from build123d import *

# Parameters (mm, degrees)
SKETCH1_W                        = 125
SKETCH1_H                        = 120
TEST_BASE_POSTION_DEPTH          = 11.215
SKETCH8_R                        = 20.5
FINGER_GEARS_DEPTH               = 7
SKETCH9_R                        = 10.5
INTERMEDIATE_GEAR_DEPTH          = 7
SKETCH11_R                       = 18.5
XL320_FINGER_KNUCKLE_MOUNT_DEPTH = 7
SKETCH10_R                       = 15.5
CONNECT_FINGER_HOLES_DEPTH       = 88.361468766
THUMB_MOUNT_HOLES_R              = 2.25
THUMB_MOUNT_HOLES_M4_DEPTH       = 88.361468766
SKETCH16_R                       = 2.25
FINGERS_MOUNT_HOLES_M4_DEPTH     = 88.361468766
SKETCH17_R                       = 3.25
CONNECT_HOLES_M6_DEPTH           = 88.361468766
NUTS_M4_DEPTH                    = 4
NUTS_M6_DEPTH                    = 6
SKETCH21_R                       = 1.5
FIX_GEAR_ROD_HOLE_DEPTH          = 2.5


with BuildPart() as part:
    # Sketch1 → Test_Base_Postion (new body)
    with BuildSketch(Plane(origin=(0, 0, 0), x_dir=(1, 0, 0), z_dir=(0, 1, 0))):
        Rectangle(SKETCH1_W, SKETCH1_H)
    extrude(amount=TEST_BASE_POSTION_DEPTH)

    # Sketch8 → Finger_Gears (cut)
    with BuildSketch(Plane(origin=(0, 11.215, 0), x_dir=(1, 0, 0), z_dir=(0, 1, 0))):
        with Locations((-25.25, -19)):
            Circle(SKETCH8_R)
        with Locations((-25.25, 19)):
            Circle(SKETCH8_R)
    extrude(amount=-FINGER_GEARS_DEPTH, mode=Mode.SUBTRACT)

    # Sketch9 → Intermediate_Gear (cut)
    with BuildSketch(Plane(origin=(0, 11.215, 0), x_dir=(1, 0, 0), z_dir=(0, 1, 0))):
        with Locations((0.646123438, -8.351488795)):
            Circle(SKETCH9_R)
    extrude(amount=-INTERMEDIATE_GEAR_DEPTH, mode=Mode.SUBTRACT)

    # Sketch11 → XL320_Finger_Knuckle_Mount (cut)
    with BuildSketch(Plane(origin=(0, 11.215, 0), x_dir=(1, 0, 0), z_dir=(0, 1, 0))):
        with Locations(Location((42, 0, 0), (0, 0, 270))):
            Circle(SKETCH11_R)
    extrude(amount=-XL320_FINGER_KNUCKLE_MOUNT_DEPTH, mode=Mode.SUBTRACT)

    # Sketch10 → Connect_Finger_Holes (cut, through all)
    with BuildSketch(Plane(origin=(0, 11.215, 0), x_dir=(1, 0, 0), z_dir=(0, 1, 0))):
        with Locations(Location((-25.25, 19, 0), (0, 0, 270))):
            Circle(SKETCH10_R)
        with Locations(Location((-25.25, -19, 0), (0, 0, 270))):
            Circle(SKETCH10_R)
        with Locations(Location((42, 0, 0), (0, 0, 270))):
            Circle(SKETCH10_R)
    extrude(amount=-CONNECT_FINGER_HOLES_DEPTH, mode=Mode.SUBTRACT)

    # Thumb_Mount_Holes → Thumb_Mount_Holes_(M4) (cut, through all)
    with BuildSketch(Plane(origin=(0, 11.215, 0), x_dir=(1, 0, 0), z_dir=(0, 1, 0))):
        with Locations(Location((21.5, 44.5, 0), (0, 0, 270))):
            Circle(THUMB_MOUNT_HOLES_R)
        with Locations(Location((42, 53.5, 0), (0, 0, 270))):
            Circle(THUMB_MOUNT_HOLES_R)
        with Locations(Location((48, -24, 0), (0, 0, 270))):
            Circle(THUMB_MOUNT_HOLES_R)
        with Locations(Location((36, -24, 0), (0, 0, 270))):
            Circle(THUMB_MOUNT_HOLES_R)
    extrude(amount=-THUMB_MOUNT_HOLES_M4_DEPTH, mode=Mode.SUBTRACT)

    # Sketch16 → Fingers_Mount_Holes_(M4) (cut, through all)
    with BuildSketch(Plane(origin=(0, 11.215, 0), x_dir=(1, 0, 0), z_dir=(0, 1, 0))):
        with Locations(Location((11.5, 41, 0), (0, 0, 270))):
            Circle(SKETCH16_R)
        with Locations(Location((11.5, -41, 0), (0, 0, 270))):
            Circle(SKETCH16_R)
        with Locations(Location((-53, 6, 0), (0, 0, 270))):
            Circle(SKETCH16_R)
        with Locations(Location((-53, -6, 0), (0, 0, 270))):
            Circle(SKETCH16_R)
    extrude(amount=-FINGERS_MOUNT_HOLES_M4_DEPTH, mode=Mode.SUBTRACT)

    # Sketch17 → Connect_Holes_(M6) (cut, through all)
    with BuildSketch(Plane(origin=(0, 11.215, 0), x_dir=(1, 0, 0), z_dir=(0, 1, 0))):
        with Locations(Location((-52.5, 50, 0), (0, 0, 270))):
            Circle(SKETCH17_R)
        with Locations(Location((-52.5, -50, 0), (0, 0, 270))):
            Circle(SKETCH17_R)
        with Locations(Location((52.5, -50, 0), (0, 0, 270))):
            Circle(SKETCH17_R)
    extrude(amount=-CONNECT_HOLES_M6_DEPTH, mode=Mode.SUBTRACT)

    # Sketch18 → Nuts_(M4) (cut)
    with BuildSketch(Plane.XZ):
        Polygon((11.5, 47.639528096), (5.75, 44.319764048), (5.75, 37.680235952), (11.5, 34.360471904), (17.25, 37.680235952), (17.25, 44.319764048), align=None)
        Polygon((11.5, -34.360471904), (5.75, -37.680235952), (5.75, -44.319764048), (11.5, -47.639528096), (17.25, -44.319764048), (17.25, -37.680235952), align=None)
        Polygon((15.75, -41.180235952), (15.75, -47.819764048), (21.5, -51.139528096), (27.25, -47.819764048), (27.25, -41.180235952), (21.5, -37.860471904), align=None)
        Polygon((42, -60.139528096), (47.75, -56.819764048), (47.75, -50.180235952), (42, -46.860471904), (36.25, -50.180235952), (36.25, -56.819764048), align=None)
    extrude(amount=-NUTS_M4_DEPTH, mode=Mode.SUBTRACT)

    # Sketch19 → Nuts_(M6) (cut)
    with BuildSketch(Plane.XZ):
        Polygon((-52.5, 58.371578903), (-59.75, 54.185789452), (-59.75, 45.814210548), (-52.5, 41.628421097), (-45.25, 45.814210548), (-45.25, 54.185789452), align=None)
        Polygon((52.5, 58.371578903), (45.25, 54.185789452), (45.25, 45.814210548), (52.5, 41.628421097), (59.75, 45.814210548), (59.75, 54.185789452), align=None)
        Polygon((-52.5, -41.628421097), (-59.75, -45.814210548), (-59.75, -54.185789452), (-52.5, -58.371578903), (-45.25, -54.185789452), (-45.25, -45.814210548), align=None)
    extrude(amount=-NUTS_M6_DEPTH, mode=Mode.SUBTRACT)

    # Sketch21 → Fix_Gear_Rod_Hole (cut)
    with BuildSketch(Plane(origin=(0, 4.215, 0), x_dir=(1, 0, 0), z_dir=(0, 1, 0))):
        with Locations(Location((0.646123438, -8.351488795, 0), (0, 0, 270))):
            Circle(SKETCH21_R)
    extrude(amount=-FIX_GEAR_ROD_HOLE_DEPTH, mode=Mode.SUBTRACT)


solid = part.part
Design review of the part built by this model. Coordinates are the model's own, in mm. A direction names the side the tool comes from. Give positions to 0.01 mm unless a question says otherwise; leave off trailing zeros. Write each loop counter-clockwise with the first axis right and the second up, starting at its lowest first coordinate (ties: lowest second). Pieces come first, ordered by that corner, then holes. Notation, with made-up numbers: M -37.5,-7.75 L -30.5,-7.75 A10 ccw -30.5,2.25 Z; hole C 39,12.5 d8. An arc over 180 degrees is marked long. Return JSON: item names as keys, results as strings. Group by question number.
Item 1: Wall thickness on line 1 along X through (y, z) = (2.25, 41); line 2 along X through (y, z) = (4, -6); line 3 along Z through (x, y) = (38, 8.5): over which ranges is each line inside the solid? List them lowest first.
Item 2: Take a section at D-D (x = -8). Give the boundary of the cut face in (y, z) (3 decimals).
Item 3: Take a section at C-C (x = 30). Give the boundary of the cut face in (y, z) (3 decimals).
Item 4: Tool access review of faces 4 (the cylindrical face through (-9.882, 2.137, 16.982)), 5 (the flat face through (42, 4, -56)): name each direction out of +Z, -Z, +X, -X, +Y, -Y from which nothing blocks a thin tool from reaching the whole face with its end or side.
Item 5: Take a section at A-A (z = 50). Give the boundary of the cut face in (x, y) (3 decimals), plus the area to 3 significant figures.
Item 6: Clearance check with a flat-ended pin moving along its axis: pin 1 Ø4.5 at (x, z) = (-50, 49.5) entering from -Y. State where the tip first meets the part, or that it passes through.
Item 7: The part is to be moulded in two halves that separate along X. For faces 1 (the flat face through (62.5, 6, 1)), 2 (the flat face through (-1, 0, -1)), 3 (the flat face through (17.25, 2, 41)), say which applies: pulls with the +X half, pulls with the -X half, needs draft (parallel to the pull), parting line crosses it, or undercut.
Item 8: Take a section at B-B (x = -25.25). Give the boundary of the cut face in (y, z) (3 decimals), plus the area to 3 significant figures.
Return value:
{
 "1": {"line 1": "x = -62.5 to 5.75, 17.25 to 62.5", "line 2": "x = -62.5 to -55.25, -50.75 to -33.69, -16.81 to 27.71, 56.29 to 62.5", "line 3": "z = -60 to -18.06, 18.06 to 22.97, 25.03 to 60"},
 "2": {"outline": "M 0,-60 L 11.215,-60 L 11.215,-30.076 L 4.215,-30.076 L 4.215,-7.924 L 11.215,-7.924 L 11.215,2.394 L 4.215,2.394 L 4.215,30.076 L 11.215,30.076 L 11.215,60 L 0,60 Z"},
 "3": {"outline": "M 0,-60 L 11.215,-60 L 11.215,-14.08 L 4.215,-14.08 L 4.215,-9.811 L 0,-9.811 Z; M 0,9.811 L 4.215,9.811 L 4.215,14.08 L 11.215,14.08 L 11.215,60 L 0,60 Z"},
 "4": {"face 4": "+Y, -Y", "face 5": "-Y"},
 "5": {"outline": "M -62.5,0 L -59.75,0 L -59.75,6 L -55.75,6 L -55.75,11.215 L -62.5,11.215 Z; M -49.25,6 L -45.25,6 L -45.25,0 L 45.25,0 L 45.25,6 L 49.25,6 L 49.25,11.215 L -49.25,11.215 Z; M 55.75,6 L 59.75,6 L 59.75,0 L 62.5,0 L 62.5,11.215 L 55.75,11.215 Z", "area": "1,160 mm2"},
 "6": {"pin 1": "stops at y = 6"},
 "7": {"face 1": "pulls with the +X half", "face 2": "needs draft", "face 3": "undercut"},
 "8": {"outline": "M 0,-60 L 11.215,-60 L 11.215,-39.5 L 4.215,-39.5 L 4.215,-34.5 L 0,-34.5 Z; M 0,-3.5 L 4.215,-3.5 L 4.215,3.5 L 0,3.5 Z; M 0,34.5 L 4.215,34.5 L 4.215,39.5 L 11.215,39.5 L 11.215,60 L 0,60 Z", "area": "531 mm2"}
}
